Verification items for the finished model (mm, model axes). Face numbers are marked on the shaded views. A direction names the side the tool comes from. Coordinates: 2 decimals unless noted, no trailing zeros. Order: outer loops, then holes, each group sorted by start corner. A loop starts at its lowest first (then second) coordinate and runs counter-clockwise, first axis right, second up. Notation, with made-up numbers: (71.5, 62.25) -> (103.5, 62.25) arc R22 cw to (103.5, 86.25) -> close; hole circle Ø3 at (-13, 87). An arc over 180 degrees is marked (long way). Use CSV: the item, a comma, the result in double quotes. Start each with the question number.
1) Sectioned sample at C-C on y = 12. Record the boundary of the cut face in (x, z), then the cut area to 3 significant figures.
2) Sectioned sample at A-A on y = 5.75. Record the boundary of the cut face in (x, z), then the cut area to 3 significant figures.
3) Sectioned sample at D-D on x = 12.5. Record the boundary of the cut face in (y, z).
4) Tool access check on the marked faces 4 and 5. Record the directions out of +Z, -Z, +X, -X, +Y, -Y that give a thin tool (end or side, any length) a straight path to the whole face; none if there is none.
5) Sectioned sample at B-B on z = 8. Record the boundary of the cut face in (x, y).
6) Go/stop test with a flat-tipped pin: pin 1 (4 mm diameter, centred on x = -11, y = -10, fed in from -Z). Record where the tip stops, or that it passes through.
7) Release check for a two-part mould opening along X. For the marked faces 1, 2 and 3 record: released by +X, released by -X, zero draft, split by the parting line, or undercut.
8) Scan lines: line 1 along X through (y, z) = (2, 22); line 2 along X through (y, z) = (10, 17.5); line 3 along Y through (x, z) = (-11, 7). Record each from-to range of solid material in increasing order.
from build123d import *

# Parameters (mm, degrees)
SKETCH_1_W          = 40
SKETCH_1_H          = 30
EXTRUDE_1_DEPTH     = 30
CUT_EXTRUDE_1_DEPTH = 43
SKETCH_3_W          = 7.285636578
SKETCH_3_H          = 18.354132306
CUT_EXTRUDE_2_DEPTH = 30


with BuildPart() as part:
    # 草圖1 → 填料-伸長1 (new body)
    with BuildSketch(Plane.XY):
        Rectangle(SKETCH_1_W, SKETCH_1_H)
    extrude(amount=EXTRUDE_1_DEPTH)

    # 草圖2 → 除料-伸長1 (cut)
    with BuildSketch(Plane.XY.offset(30)):
        Polygon((10, 15), (20, 5), (20, 15), align=None)
    extrude(amount=-CUT_EXTRUDE_1_DEPTH, mode=Mode.SUBTRACT)

    # 草圖3 → 除料-伸長2 (cut)
    with BuildSketch(Plane.XY.offset(30)):
        with Locations((-8.642818289, 5.822933847)):
            Rectangle(SKETCH_3_W, SKETCH_3_H)
    extrude(amount=-CUT_EXTRUDE_2_DEPTH, mode=Mode.SUBTRACT)


solid = part.part
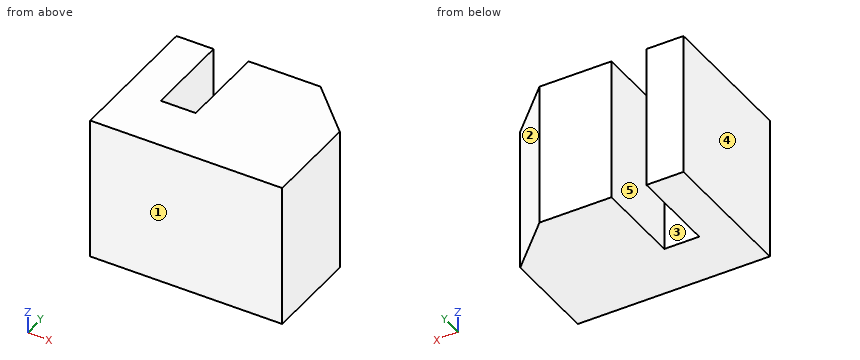
Answers follow:
1,outline,"(-20, 0) -> (-12.29, 0) -> (-12.29, 30) -> (-20, 30) -> close; (-5, 0) -> (13, 0) -> (13, 30) -> (-5, 30) -> close"
1,area,"771 mm²"
2,outline,"(-20, 0) -> (-12.29, 0) -> (-12.29, 30) -> (-20, 30) -> close; (-5, 0) -> (19.25, 0) -> (19.25, 30) -> (-5, 30) -> close"
2,area,"959 mm²"
3,outline,"(-15, 0) -> (12.5, 0) -> (12.5, 30) -> (-15, 30) -> close"
4,face 4,"+Z, -Z, -X, +Y, -Y"
4,face 5,"+Z, -Z, +Y"
5,outline,"(-20, -15) -> (20, -15) -> (20, 5) -> (10, 15) -> (-5, 15) -> (-5, -3.35) -> (-12.29, -3.35) -> (-12.29, 15) -> (-20, 15) -> close"
6,pin 1,"stops at z = 0"
7,face 1,"zero draft"
7,face 2,"released by +X"
7,face 3,"undercut"
8,line 1,"x = -20 to -12.29, -5 to 20"
8,line 2,"x = -20 to -12.29, -5 to 15"
8,line 3,"y = -15 to -3.35"
